Autodesk Fusion 360 part; units mm, degrees
sketch "Sketch1" plane through (0, 0, 0) normal (0, 0, 1) x (1, 0, 0)
  circle A0 centre (0, 0) radius 10.5
  circle A1 centre (0, 0) radius 4
  arc A2 (11.8123, 44.4575) -> (-44.4575, -11.8123) centre (0, 0) ccw
  arc A3 (14.1876, 53.3973) -> (-53.3973, -14.1876) centre (0, 0) ccw
  arc A4 (-53.3973, -14.1876) -> (-44.4575, -11.8123) centre (-48.9274, -13) ccw
  arc A5 (11.8123, 44.4575) -> (14.1876, 53.3973) centre (13, 48.9274) ccw
  line L0 (25, 58.0996) -> (25, -65)
  line L1 (-63.25, -65) -> (25, -65)
  line L2 (-63.25, 0) -> (-63.25, -65)
  arc A6 (25, 58.0996) -> (-63.25, 0) centre (0, 0) ccw
  circle A7 centre (-51.25, -50) radius 3
  circle A8 centre (-19.125, -50) radius 3
  circle A9 centre (8, -50) radius 3
  dimension "d1" = 21
  dimension "d2" = 8
  dimension "d3" = 92
  dimension "d4" = 110.5
  dimension "d5" = 9.25
  dimension "d6" = 9.25
  dimension "d9" = 126.5
  dimension "d10" = 25
  dimension "d11" = 12
  dimension "d13" = 6
  dimension "d14" = 6
  dimension "d15" = 6
  dimension "d16" = 15
  dimension "d18" = 15
  dimension "d19" = 15
  dimension "d21" = 12
  dimension "d22" = 17
  dimension "d29" = 65
  dimension "d30" = 50.625
  dimension "d33" = 44.125
  dimension "d34" = 13
extrude "Extrude1" add sketch "Sketch1" along normal blind 8 contours L0 L1 L2 A6
fillet "Fillet1" radius 12 3 edges at (-63.25, -65, 4) (25, -65, 4) (25, 58.0996, 4)
equation "d4 = d3 + 18.5 mm"
equation "d5 = d6"
equation "d6 = ( d4 - d3 ) / 2"
equation "d9 = d4 + 16 mm"
equation "d18 = d16"
equation "d19 = d16"
equation "d21 = d11"
equation "d22 = d11 + 5 mm"
equation "d33 = ( ( d9 / 2 ) + d10 ) / 2"
equation "d34 = d10 - d11"
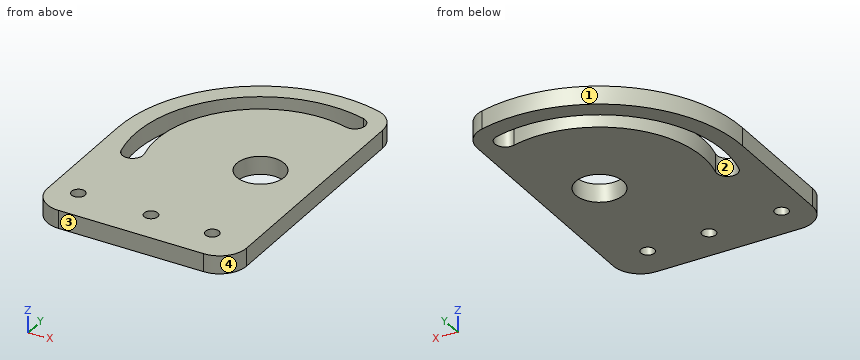
Can you work these out from the model? Positions are in its coordinate system, mm. Face numbers are marked on the shaded views. Coordinates: 2 decimals unless noted, no trailing zeros. Write each loop counter-clockwise with the first axis right and the second up, starting at its lowest first coordinate (ties: lowest second). Pieces come first, ordered by that corner, then holes. Notation, with made-up numbers: (89.25, -8.75) -> (99.25, -8.75) arc R30 cw to (99.25, 21.25) -> close; hole circle Ø2 at (-7, 37). An arc over 180 degrees is marked (long way). Write item = value, one per line.
(1) Imagine slicing it at D-D (x = 8). Please give me the cut outline in (y, z).
Verdict:
outline = (-65, 0) -> (-53, 0) -> (-53, 8) -> (-65, 8) -> close; (-47, 0) -> (-6.8, 0) -> (-6.8, 8) -> (-47, 8) -> close; (6.8, 0) -> (45.3, 0) -> (45.3, 8) -> (6.8, 8) -> close; (54.67, 0) -> (62.74, 0) -> (62.74, 8) -> (54.67, 8) -> close
(2) Imagine slicing it at A-A (y = -50). Please give me the cut outline in (x, z) (3 decimals), and give its area (3 significant figures).
Verdict:
outline = (-63.25, 0) -> (-54.25, 0) -> (-54.25, 8) -> (-63.25, 8) -> close; (-48.25, 0) -> (-22.125, 0) -> (-22.125, 8) -> (-48.25, 8) -> close; (-16.125, 0) -> (5, 0) -> (5, 8) -> (-16.125, 8) -> close; (11, 0) -> (25, 0) -> (25, 8) -> (11, 8) -> close
area = 562 mm^2
(3) If I drill on probe 1 along Y at (x, z) = (0, 4.25); probe 2 along X at (y, z) = (1.5, 3); probe 3 along Y at (x, z) = (8, 3.5), over which ranges is the centre line in solid material (lowest first)?
Verdict:
probe_1 = -65 to -10.5, 10.5 to 46, 55.25 to 63.25
probe_2 = -63.23 to -55.23, -45.98 to -10.39, 10.39 to 25
probe_3 = -65 to -53, -47 to -6.8, 6.8 to 45.3, 54.67 to 62.74
(4) For pin 1 (1.5 mm diameter, centred on x = -16, z = 3.5, fed in from +Y); pin 2 (5.5 mm diameter, centred on x = -19.125, y = -50, fed in from +Z); pin 3 (3 mm diameter, centred on y = 37, z = 3, fed in from -X), each with a flat end and sliding along its axis, tell me the tip position at first contact or that it passes through.
Verdict:
pin_1 = 61.38
pin_2 = through
pin_3 = -52.35
(5) Thinking about a two-plate mould opening in X: for the marked faces 1, 2, 3 and 4, which applies, +X half, -X half, draft (parallel to the pull), parting line (faces both ways), or undercut?
Verdict:
face_1 = parting line
face_2 = undercut
face_3 = draft
face_4 = +X half
(6) Imagine slicing it at C-C (y = 6). Please give me the cut outline in (x, z), and give its area (3 significant figures).
Verdict:
outline = (-62.96, 0) -> (-54.92, 0) -> (-54.92, 8) -> (-62.96, 8) -> close; (-45.61, 0) -> (-8.62, 0) -> (-8.62, 8) -> (-45.61, 8) -> close; (8.62, 0) -> (25, 0) -> (25, 8) -> (8.62, 8) -> close
area = 491 mm^2
(7) Imagine slicing it at B-B (x = -14). Please give me the cut outline in (y, z).
Verdict:
outline = (-65, 0) -> (43.82, 0) -> (43.82, 8) -> (-65, 8) -> close; (53.45, 0) -> (61.68, 0) -> (61.68, 8) -> (53.45, 8) -> close
